Geometry check sheet. Reference: drawing and pictorial views, mm from the part's lowest x, y, z. Round coordinates to 2 decimals unless told otherwise and drop trailing zeros. Loops run counter-clockwise (first coordinate to the right, second up) from the corner with the lowest first, then second, coordinate; pieces in that order, holes last. Notation, with made-up numbers: (79, -27) - (83, -27) arc R15 cw to (83, -8) - close; hole circle Ø8 at (13, -6). An arc over 180 degrees is marked (long way). Return JSON: item names as keys, results as strings.
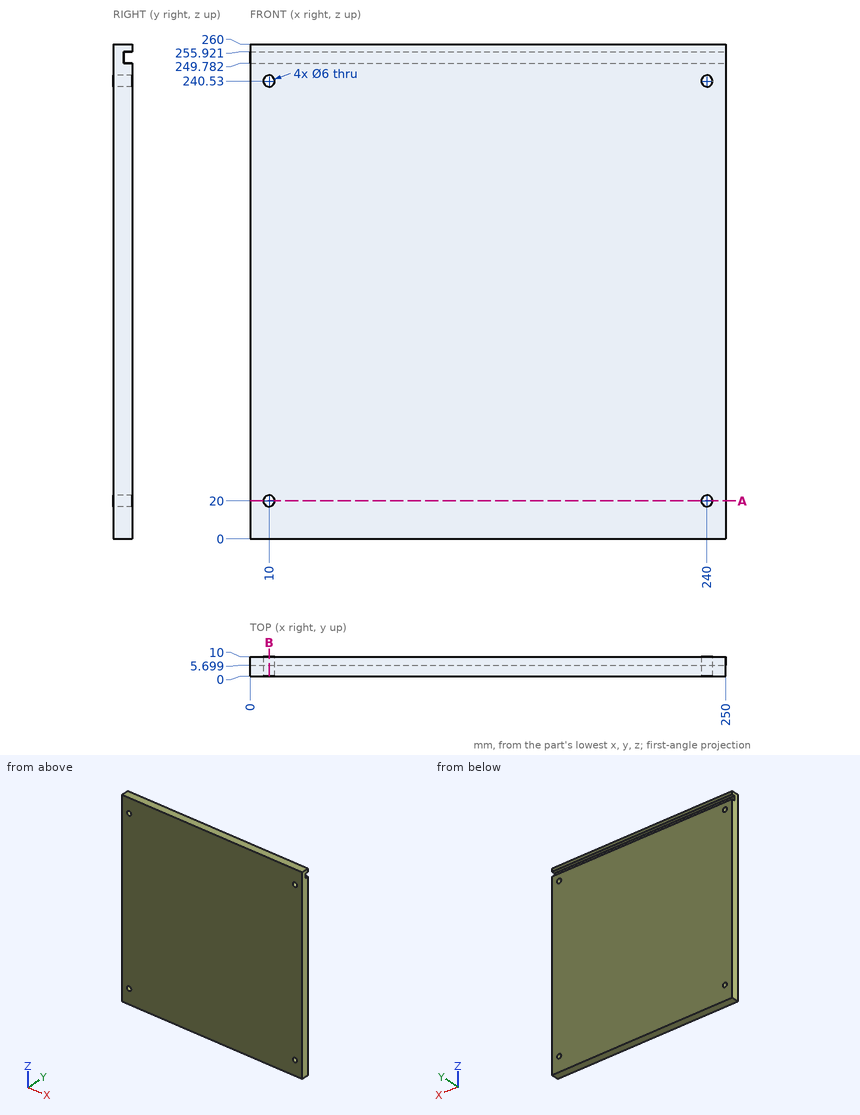
Q1. Scan lines: probe 1 along Z at (x, y) = (10, 7.25); probe 2 along X at (y, z) = (3.75, 20); probe 3 along Z at (x, y) = (240, 4.5). Record each from-to range of solid material in increasing order. Write a range as [from, to].
Answer key:
{"probe 1": "z = [0, 17], [23, 237.53], [243.53, 249.78], [255.92, 260]", "probe 2": "x = [0, 7], [13, 237], [243, 250]", "probe 3": "z = [0, 17], [23, 237.53], [243.53, 260]"}
Q2. Sectioned sample at A-A (z = 20). Enter the section's corners in (x, y).
Answer key:
{"outline": "(0, 0) - (7, 0) - (7, 10) - (0, 10) - close; (13, 0) - (237, 0) - (237, 10) - (13, 10) - close; (243, 0) - (250, 0) - (250, 10) - (243, 10) - close"}
Q3. Sectioned sample at B-B (x = 10). Enter the section's corners in (y, z), plus the area to 3 significant figures.
Answer key:
{"outline": "(0, 0) - (10, 0) - (10, 17) - (0, 17) - close; (0, 23) - (10, 23) - (10, 237.53) - (0, 237.53) - close; (0, 243.53) - (10, 243.53) - (10, 249.78) - (5.7, 249.78) - (5.7, 255.92) - (10, 255.92) - (10, 260) - (0, 260) - close", "area": "2,450 mm²"}
Q4. Depth check by flat-ended pin: P1, Ø1.8, axis at x = 111, z = 253.5, coming from the +Y side. Enter the tip coordinate at first touch or a pass-through.
Answer key:
{"P1": "stops at y = 5.7"}
